Autodesk Inventor part; units mm, degrees
ref_plane "YZ Plane" through (0, 0, 0) normal (1, 0, 0) x (0, 1, 0)
ref_plane "XZ Plane" through (0, 0, 0) normal (0, 1, 0) x (-1, 0, 0)
ref_plane "XY Plane" through (0, 0, 0) normal (0, 0, 1) x (1, 0, 0)
sketch "Sketch1" plane through (0, 0, 0) normal (0, 0, 1) x (1, 0, 0)
  line L0 (-21.5469, -17.0285) -> (21.5469, -17.0285)
  line L1 (21.5469, -17.0285) -> (21.5469, 17.0285)
  line L2 (21.5469, 17.0285) -> (-21.5469, 17.0285)
  line L3 (-21.5469, 17.0285) -> (-21.5469, -17.0285)
extrude "Extrusion1" add sketch "Sketch1" along normal blind 7.62
fillet "Fillet1" radius 5.08 8 edges at (-21.5469, -17.0285, 3.81) (-21.5469, 0, 7.62) (-21.5469, 17.0285, 3.81) (21.5469, 17.0285, 3.81) (21.5469, -17.0285, 3.81) (0, -17.0285, 7.62) (21.5469, 0, 7.62) (0, 17.0285, 7.62)
shell "Shell1" thickness 2.54 removed faces 1 at (5.489, -5.6762, 0)
properties part number "Adaptive Lid"
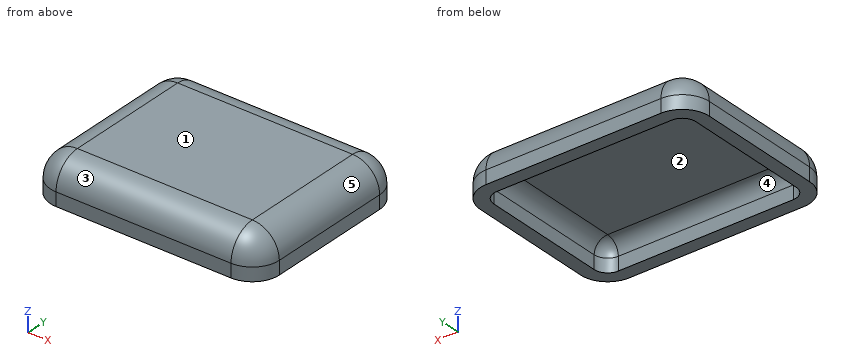
Work out the finished part from the listing and answer in its coordinate system (mm). Face numbers are marked on the shaded views. A direction names the side the tool comes from. Give positions to 0.01 mm unless a question says otherwise; leave off trailing zeros. Write each loop counter-clockwise with the first axis right and the second up, starting at its lowest first coordinate (ties: lowest second). Pieces come first, ordered by that corner, then holes.
(1) Which of the six approach directions +Z, -Z, +X, -X, +Y, -Y give full straight-line access (tool end or side, diameter ignored) to the marked faces 1 and 2?
Final values:
face 1: +Z, +X, -X, +Y, -Y
face 2: -Z
(2) Straight lines are drawn through the part: line 1 (X direction, y = 4, z = 1.5); line 2 (Z direction, x = -9, y = 4.5); line 3 (Y direction, x = -16.5, z = 2). For each, find the intervals that lie inside material, in ascending order.
Final values:
line 1: x = -21.55 to -19.01, 19.01 to 21.55
line 2: z = 5.08 to 7.62
line 3: y = -17.03 to -14.49, 14.49 to 17.03
(3) The mould has two halves that part along X. Classify the marked faces 3, 4 and 5: pulls with the +X half, pulls with the -X half, needs draft (parallel to the pull), parting line crosses it, or undercut.
Final values:
face 3: needs draft
face 4: undercut
face 5: pulls with the +X half
(4) The part is cut by section A-A on z = 1.5. Write down the section's boundary in (x, y).
Final values:
outline: (-21.55, -11.95) arc R5.08 ccw to (-16.47, -17.03) - (16.47, -17.03) arc R5.08 ccw to (21.55, -11.95) - (21.55, 11.95) arc R5.08 ccw to (16.47, 17.03) - (-16.47, 17.03) arc R5.08 ccw to (-21.55, 11.95) - close; hole (-19.01, -11.95) arc R2.54 ccw to (-16.47, -14.49) - (16.47, -14.49) arc R2.54 ccw to (19.01, -11.95) - (19.01, 11.95) arc R2.54 ccw to (16.47, 14.49) - (-16.47, 14.49) arc R2.54 ccw to (-19.01, 11.95) - close
(5) The part is cut by section C-C on y = -3. Write down the section's boundary in (x, z), plus the area to 3 significant figures.
Final values:
outline: (-21.55, 0) - (-19.01, 0) - (-19.01, 2.54) arc R2.54 cw to (-16.47, 5.08) - (16.47, 5.08) arc R2.54 cw to (19.01, 2.54) - (19.01, 0) - (21.55, 0) - (21.55, 2.54) arc R5.08 ccw to (16.47, 7.62) - (-16.47, 7.62) arc R5.08 ccw to (-21.55, 2.54) - close
area: 127 mm2
(6) The part is cut by section B-B on x = -13.5. Write down the section's boundary in (y, z).
Final values:
outline: (-17.03, 0) - (-14.49, 0) - (-14.49, 2.54) arc R2.54 cw to (-11.95, 5.08) - (11.95, 5.08) arc R2.54 cw to (14.49, 2.54) - (14.49, 0) - (17.03, 0) - (17.03, 2.54) arc R5.08 ccw to (11.95, 7.62) - (-11.95, 7.62) arc R5.08 ccw to (-17.03, 2.54) - close
(7) Flat-ended cylindrical pins translate along their axes: pin 1 Ø1 at (x, z) = (0.5, 3.5) entering from +Y; pin 2 Ø19 at (x, y) = (4, 1) entering from -Z. Find the tip coordinate at first contact, or state that the pin passes through.
Final values:
pin 1: stops at y = 17.01
pin 2: stops at z = 5.08
(8) The part is cut by section D-D on z = 7. Write down the section's boundary in (x, y).
Final values:
outline: (-18.9, -11.95) arc R2.43 ccw to (-16.47, -14.38) - (16.47, -14.38) arc R2.43 ccw to (18.9, -11.95) - (18.9, 11.95) arc R2.43 ccw to (16.47, 14.38) - (-16.47, 14.38) arc R2.43 ccw to (-18.9, 11.95) - close
